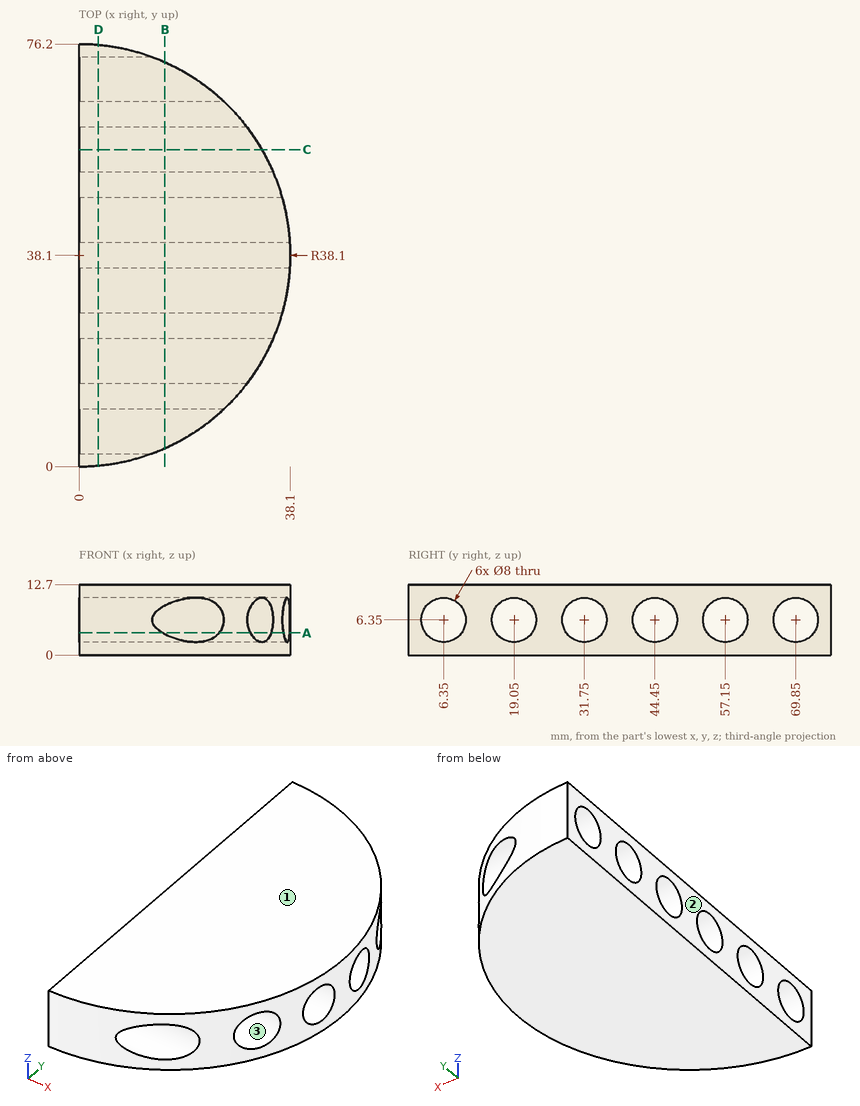
Verification items for this drawing (mm, ordinates from the low corner). Give positions to 0.01 mm unless a question says otherwise; leave off trailing zeros. Write each loop counter-clockwise with the first axis right and the second up, starting at its lowest first coordinate (ties: lowest second). Pieces come first, ordered by that corner, then holes. Notation, with made-up numbers: (-2.75, 11) - (45.25, 11) arc R15 ccw to (45.25, 40) - close; hole circle Ø11 at (42.5, 68). An arc over 180 degrees is marked (long way). Answer as a JSON object with one key per item and string values. Group by question number.
1) Sectioned sample at C-C (y = 57.15). Record the cut outline in (x, z).
2) Sectioned sample at B-B (x = 15.5). Record the cut outline in (y, z).
3) Sectioned sample at A-A (z = 4). Record the cut outline in (x, y).
4) Depth check by flat-ended pin: P1, Ø6, axis at x = 11.5, z = 3.5, coming from the +Y side; P2, Ø6, axis at y = 27.5, z = 4, coming from the +X side. Enter the tip coordinate at first touch or a pass-through.
5) Sectioned sample at D-D (x = 3.5). Record the cut outline in (y, z), then the cut area to 3 significant figures.
6) Release check for a two-part mould opening along Z. For the marked faces 1, 2 and 3 record: pulls with the +Z half, pulls with the -Z half, needs draft (parallel to the pull), parting line crosses it, or undercut.
7) Thickness scan on probe 1 along Z at (x, y) = (7, 6); probe 2 along Y at (x, z) = (26.5, 3.5); probe 3 along Y at (x, z) = (23, 3). Record the ranges inside material, lowest first. Write a range as from..to.
Geometry results:
{
 "1": {"outline": "(0, 0) - (33, 0) - (33, 2.35) - (0, 2.35) - close; (0, 10.35) - (33, 10.35) - (33, 12.7) - (0, 12.7) - close"},
 "2": {"outline": "(3.3, 0) - (72.9, 0) - (72.9, 3.77) arc R4 cw (long way) to (72.9, 8.93) - (72.9, 12.7) - (3.3, 12.7) - (3.3, 8.93) arc R4 cw (long way) to (3.3, 3.77) - close; hole circle Ø8 at (19.05, 6.35); hole circle Ø8 at (31.75, 6.35); hole circle Ø8 at (44.45, 6.35); hole circle Ø8 at (57.15, 6.35)"},
 "3": {"outline": "(0, 0) arc R38.1 ccw to (15.08, 3.11) - (0, 3.11) - close; (0, 9.59) - (25.27, 9.59) arc R38.1 ccw to (30.9, 15.81) - (0, 15.81) - close; (0, 22.29) - (34.66, 22.29) arc R38.1 ccw to (36.87, 28.51) - (0, 28.51) - close; (0, 34.99) - (37.97, 34.99) arc R38.1 ccw to (37.97, 41.21) - (0, 41.21) - close; (0, 47.69) - (36.87, 47.69) arc R38.1 ccw to (34.66, 53.91) - (0, 53.91) - close; (0, 60.39) - (30.9, 60.39) arc R38.1 ccw to (25.27, 66.61) - (0, 66.61) - close; (0, 73.09) - (15.08, 73.09) arc R38.1 ccw to (0, 76.2) - close"},
 "4": {"P1": "stops at y = 75.24", "P2": "stops at x = 37.27"},
 "5": {"outline": "(0.16, 0) - (76.04, 0) - (76.04, 12.7) - (0.16, 12.7) - close; hole circle Ø8 at (6.35, 6.35); hole circle Ø8 at (19.05, 6.35); hole circle Ø8 at (31.75, 6.35); hole circle Ø8 at (44.45, 6.35); hole circle Ø8 at (57.15, 6.35); hole circle Ø8 at (69.85, 6.35)", "area": "662 mm^2"},
 "6": {"face 1": "pulls with the +Z half", "face 2": "needs draft", "face 3": "undercut"},
 "7": {"probe 1": "z = 0..2.37, 10.33..12.7", "probe 2": "y = 10.73..16.24, 21.86..28.94, 34.56..41.64, 47.26..54.34, 59.96..65.47", "probe 3": "y = 8.54..16.86, 21.24..29.56, 33.94..42.26, 46.64..54.96, 59.34..67.66"}
}
